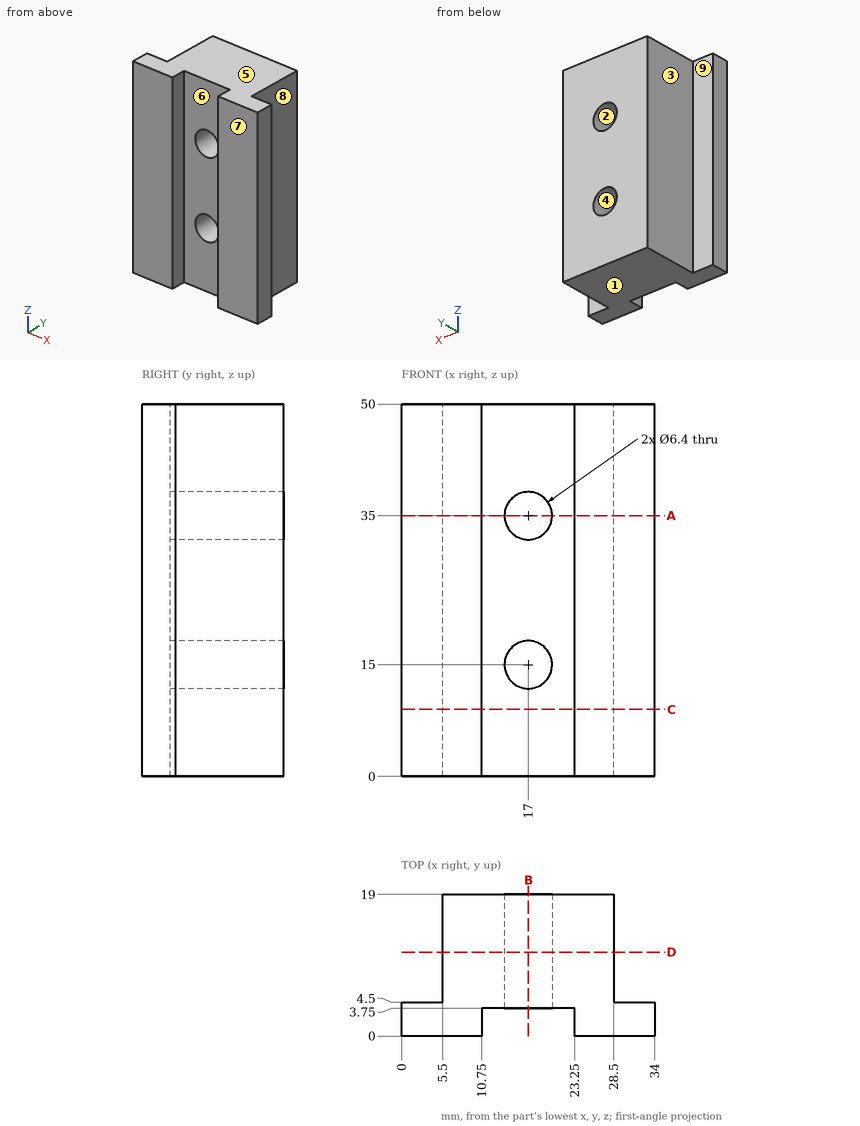
Source: three-view drawing plus pictorial views. Frame: mm from the lowest corner of the part. A direction names the side the tool comes from. Give positions to 0.01 mm unless a question says otherwise; leave off trailing zeros. Order: outer loops, then holes, each group sorted by start corner. A loop starts at its lowest first (then second) coordinate and runs counter-clockwise, first axis right, second up.
1. Section D-D on y = 11.25. Return the cut outline in (x, z), and give its area (3 significant figures).
Derived:
outline: (5.5, 0) - (28.5, 0) - (28.5, 50) - (5.5, 50) - close; hole circle Ø6.4 at (17, 15); hole circle Ø6.4 at (17, 35)
area: 1,090 mm2
2. Reachability of the marked faces 5, 6, 7, 8 and 9 from +Z, -Z, +X, -X, +Y, -Y: full face, straight path, thin tool, end or side. Return the list, or none.
Derived:
face 5: +Z, +X, -X, +Y, -Y
face 6: +Z, -Z, -Y
face 7: +Z, -Z, +X, -X, -Y
face 8: +Z, -Z, +X, +Y
face 9: +Z, -Z, -X, +Y
3. Pin query (flat end, axial travel): pin 1 (10 mm diameter, centred on x = 16.5, z = 14, fed in from -Y); pin 2 (5 mm diameter, centred on x = 17, z = 35, fed in from -Y); pin 3 (4.5 mm diameter, centred on y = 8.5, z = 15.5, fed in from +X); pin 4 (4.5 mm diameter, centred on x = 2.5, z = 20.5, fed in from +Y). Return the tip coordinate at first contact, or that it passes through.
Derived:
pin 1: stops at y = 3.75
pin 2: passes through
pin 3: stops at x = 28.5
pin 4: stops at y = 4.5
4. Section B-B on x = 17. Return the cut outline in (y, z), and give its area (3 significant figures).
Derived:
outline: (3.75, 0) - (19, 0) - (19, 11.8) - (3.75, 11.8) - close; (3.75, 18.2) - (19, 18.2) - (19, 31.8) - (3.75, 31.8) - close; (3.75, 38.2) - (19, 38.2) - (19, 50) - (3.75, 50) - close
area: 567 mm2
5. Material intervals for L1, parallel to X at y = 7.75, z = 35; L2, parallel to X at y = 2.5, z = 15.5; L3, parallel to Z at x = 18.5, y = 4, sorted ascending.
Derived:
L1: x = 5.5 to 13.8, 20.2 to 28.5
L2: x = 0 to 10.75, 23.25 to 34
L3: z = 0 to 12.17, 17.83 to 32.17, 37.83 to 50
6. Section A-A on z = 35. Return the cut outline in (x, y).
Derived:
outline: (0, 0) - (10.75, 0) - (10.75, 3.75) - (13.8, 3.75) - (13.8, 19) - (5.5, 19) - (5.5, 4.5) - (0, 4.5) - close; (20.2, 3.75) - (23.25, 3.75) - (23.25, 0) - (34, 0) - (34, 4.5) - (28.5, 4.5) - (28.5, 19) - (20.2, 19) - close
7. Mould query, pull axis Z, two halves, no side actions, for the marked faces 1, 2, 3 and 4. Classes: released by +Z, released by -Z, zero draft, split by the parting line, or undercut.
Derived:
face 1: released by -Z
face 2: undercut
face 3: zero draft
face 4: undercut
8. Section C-C on z = 9. Return the cut outline in (x, y).
Derived:
outline: (0, 0) - (10.75, 0) - (10.75, 3.75) - (23.25, 3.75) - (23.25, 0) - (34, 0) - (34, 4.5) - (28.5, 4.5) - (28.5, 19) - (5.5, 19) - (5.5, 4.5) - (0, 4.5) - close
